Geometry: see drawing. Coordinates: mm, zero at the bounding-box minimum. A direction names the side the tool comes from. Coordinates: 2 decimals unless noted, no trailing zeros. Write each loop counter-clockwise with the first axis right and the second up, starting at its lowest first coordinate (ties: lowest second). Pieces come first, ordered by that corner, then holes. Notation, with made-up numbers: (56.5, 60) - (106.5, 60) arc R11 cw to (106.5, 75) - close; hole circle Ø4 at (85, 60). An arc over 180 degrees is marked (long way). One line per question, with ' | ' between items. Start each with the question number.
Q1. Line query: line 1 (X direction, y = 5.5, z = 30); line 2 (Y direction, x = 42, z = 52); line 3 (Y direction, x = 45, z = 24). Output: solid intervals per line, ascending.
Q2. Cut plane C-C, the plane y = 16.25. Return loops of the section in (x, z), plus the area to 3 significant figures.
Q3. Access query for the marked faces 4 and 5. Directions: +Z, -Z, +X, -X, +Y, -Y. A direction counts if a zero-diameter tool reaches every point of the face in a straight line with its end or side. Return the directions, or none.
Q4. Cut plane A-A, the plane x = 30. Return loops of the section in (y, z), plus the area to 3 significant figures.
Q5. Cut plane D-D, the plane x = 56. Return loops of the section in (y, z).
Q6. Cut plane B-B, the plane z = 30. Return loops of the section in (x, y).
Q7. Contact query for flat-ended pins moving along their axis: P1, Ø3, axis at x = 8.5, y = 4, coming from the -Z side; P2, Ø8, axis at y = 16.5, z = 35, coming from the +X side; P3, Ø4, axis at x = 19.5, z = 37.5, coming from the +Y side; P4, Ø1.5, axis at y = 15.5, z = 38, coming from the -X side. Output: stop coordinate, or through.
Q8. Draft query along Z for the marked faces 1, 2 and 3. Return one class per face: +Z half, -Z half, draft (parallel to the pull), parting line (faces both ways), or undercut.
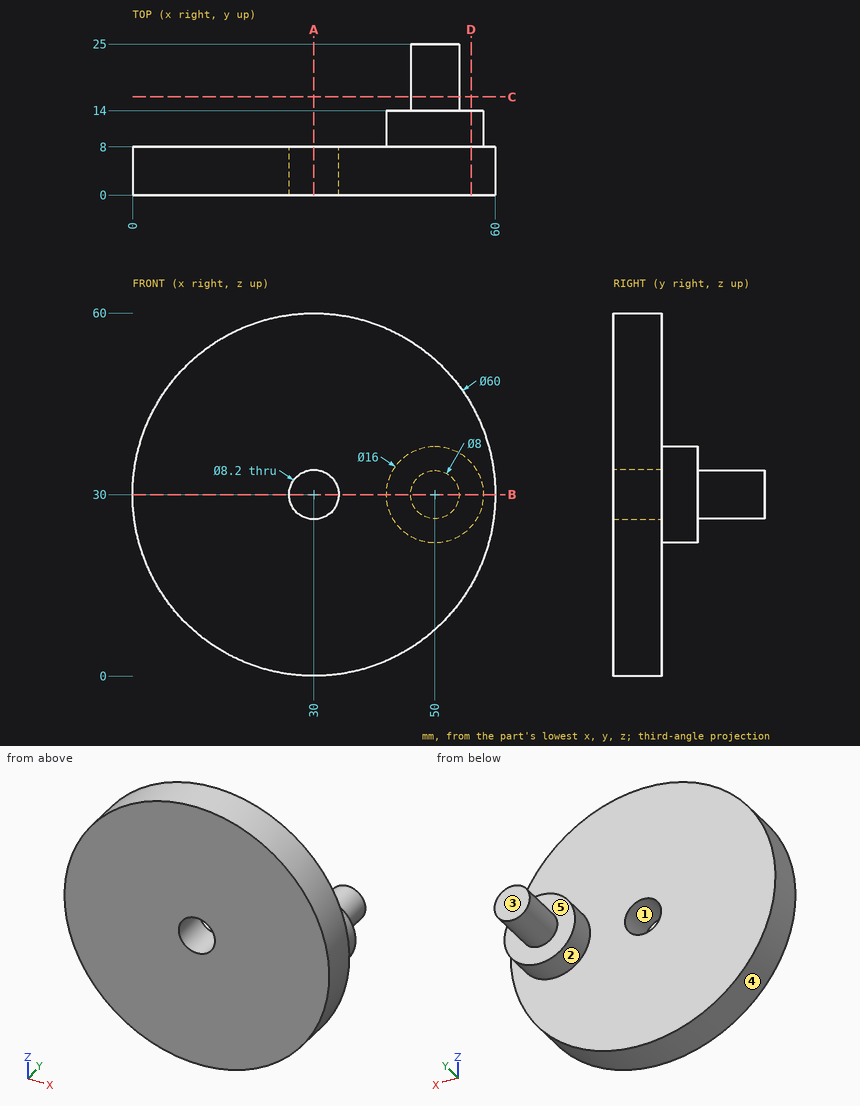
Reply:
1) line 1: x = 0 to 25.9, 34.1 to 60 | line 2: y = 0 to 8 | line 3: y = 0 to 14
2) outline: circle Ø8 at (50, 30) | area: 50.3 mm^2
3) face 4: +Y, -Y | face 5: +Y
4) outline: (0, 0) - (8, 0) - (8, 25.9) - (0, 25.9) - close; (0, 34.1) - (8, 34.1) - (8, 60) - (0, 60) - close | area: 414 mm^2
5) outline: (0, 15.03) - (8, 15.03) - (8, 24.71) - (14, 24.71) - (14, 35.29) - (8, 35.29) - (8, 44.97) - (0, 44.97) - close
6) outline: (0, 0) - (25.9, 0) - (25.9, 8) - (0, 8) - close; (34.1, 0) - (60, 0) - (60, 8) - (58, 8) - (58, 14) - (54, 14) - (54, 25) - (46, 25) - (46, 14) - (42, 14) - (42, 8) - (34.1, 8) - close
7) P1: stops at z = 7.64 | P2: stops at x = 57.78 | P3: stops at y = 8 | P4: passes through
8) face 1: undercut | face 2: parting line | face 3: draft
